Check sheet for the modelled part. Datum: model origin and axes. Units: mm. A direction names the side the tool comes from. Round coordinates to 2 decimals unless told otherwise and drop trailing zeros. Loops run counter-clockwise (first coordinate to the right, second up) from the corner with the lowest first, then second, coordinate; pieces in that order, holes last. Notation, with made-up numbers: (-2.75, -32.5) - (54.25, -32.5) arc R18 cw to (54.25, 1.5) - close; hole circle Ø2 at (2.25, 16). An arc over 180 degrees is marked (long way). Answer in a Markdown table with one row per item. Add a question column.
(1) Thickness scan on line 1 along X through (y, z) = (-49.5, 72.5); line 2 along Z through (x, y) = (5.25, -86); line 3 along Z through (x, y) = (19.5, -26.5). Record the ranges inside material, lowest first.
(2) Cross-section at C-C on z = 62. Enter the section's corners in (x, y).
(3) Cross-section at B-B on x = 8.5. Enter the section's corners in (y, z), then the cut area to 3 significant figures.
(4) Cross-section at A-A on y = -59. Enter the section's corners in (x, z).
(5) Access from +Z, -Z, +X, -X, +Y, -Y to the whole of each face (thin tool, end or side, straight path). Record for faces 1 (the flat face through (0, -52, -2)), 2 (the flat face through (12.14, -56.25, 61.24)), 3 (the flat face through (12.14, -54.114, 74.731)), 4 (the flat face through (21.799, -49, 67)), 5 (the flat face through (12.14, -40.84, 72.44)).
(6) Gauge pin test, flat ends, axial feed: pin 1 (1 mm diameter, centred on x = 18.5, z = 55.5, fed in from -Y); pin 2 (7.5 mm diameter, centred on x = 8, y = -82.5, fed in from +Z); pin 3 (1 mm diameter, centred on x = 6.5, z = 15, fed in from +Y). Record the tip position at first contact, or that the pin passes through.
(7) Cross-section at D-D on y = -85. Enter the section's corners in (x, z), then the cut area to 3 significant figures.
(8) Mould release check, pull along Z, two halves, no side actions. Record for faces 6 (the flat face through (2.749, -49, 67)), 7 (the flat face through (12.52, -12.79, 35.32)), 8 (the flat face through (13, -76, 0)): +Z half, -Z half, draft (parallel to the pull), parting line (faces both ways), or undercut.
from build123d import *

# Parameters (mm, degrees)
F1_DEPTH = 25.4
F2_W     = 19.05
F2_H     = 19.05
F3_DEPTH = 19.05


with BuildPart() as f1:
    # F0 (on Right) → F1 (new body)
    with BuildSketch(Plane.YZ):
        Polygon((-67.0450606095, 41.7946282453), (-51.9119330465, 0), (0, 0), (-25.9425043938, 71.6479341348), align=None)
        Polygon((-51.9119330465, 0), (-101.6, 0), (-101.6, -50.8), (0, -50.8), (0, 0), align=None)
    extrude(amount=F1_DEPTH)

    # F2 (on face) → F3 (join)
    with BuildSketch(Plane(origin=(0, -43.0264861608, 59.2396223299), x_dir=(1, 0, 0), z_dir=(0, -0.5876635018, 0.8091054373))):
        with Locations((12.2738424689, 0)):
            Rectangle(F2_W, F2_H)
    extrude(amount=F3_DEPTH)


solid = f1.part
Answers:
| question | item | result |
|---|---|---|
| 1 | line 1 | x = 2.75 to 21.8 |
| 1 | line 2 | z = -50.8 to 0 |
| 1 | line 3 | z = -50.8 to 71.24 |
| 2 | outline | (0, -39.23) - (2.75, -39.23) - (2.75, -56.8) - (21.8, -56.8) - (21.8, -39.23) - (25.4, -39.23) - (25.4, -22.45) - (0, -22.45) - close |
| 3 | outline | (-101.6, -50.8) - (0, -50.8) - (0, 0) - (-25.94, 71.65) - (-35.32, 64.84) - (-46.51, 80.25) - (-61.93, 69.06) - (-50.73, 53.64) - (-67.05, 41.79) - (-51.91, 0) - (-101.6, 0) - close |
| 3 | area | 8,470 mm^2 |
| 4 | outline | (0, -50.8) - (25.4, -50.8) - (25.4, 0) - (0, 0) - close; (0, 19.58) - (25.4, 19.58) - (25.4, 47.64) - (0, 47.64) - close; (2.75, 65.02) - (21.8, 65.02) - (21.8, 71.18) - (2.75, 71.18) - close |
| 5 | face 1 | +Z, -Z, -X, +Y, -Y |
| 5 | face 2 | +X, -X, -Y |
| 5 | face 3 | +Z, +X, -X, -Y |
| 5 | face 4 | +Z, +X, -Y |
| 5 | face 5 | +Z, +X, -X |
| 6 | pin 1 | stops at y = -52.45 |
| 6 | pin 2 | stops at z = 0 |
| 6 | pin 3 | stops at y = -5.25 |
| 7 | outline | (0, -50.8) - (25.4, -50.8) - (25.4, 0) - (0, 0) - close |
| 7 | area | 1,290 mm^2 |
| 8 | face 6 | draft |
| 8 | face 7 | +Z half |
| 8 | face 8 | undercut |
